Could you check a few things on this model? Use its own coordinates, in mm. Face numbers are marked on the shaded views. A direction names the side the tool comes from. Give positions to 0.01 mm unless a question says otherwise; leave off trailing zeros. Order: outer loops, then holes, each group sorted by start corner. A loop starts at its lowest first (then second) coordinate and runs counter-clockwise, first axis right, second up. Notation, with made-up numbers: (-38, 69) -> (-17, 69) arc R12 ccw to (-17, 83) -> close; hole circle Ø6 at (72, 45). An arc over 180 degrees is marked (long way). One line per item, written item: value.
```python
from build123d import *

# Parameters (mm, degrees)
ESQUISSE1_R                  = 20
EXTRUSION1_DEPTH             = 10.8
ESQUISSE2_R                  = 12
EXTRUSION2_DEPTH             = 15.7
ESQUISSE3_R                  = 11
EXTRUSION3_DEPTH             = 18
CHANFREIN1_SIZE              = 1
CHANFREIN1_OF_SYM_TRIE2_SIZE = 1


with BuildPart() as part:
    # Esquisse1 → Extrusion1 (new, symmetric)
    with BuildSketch(Plane.XY):
        with Locations(Location((0, 0, 0), (0, 0, 180))):
            Circle(ESQUISSE1_R)
    extrude(amount=EXTRUSION1_DEPTH, both=True)

    # Esquisse2 → Extrusion2 (add)
    with BuildSketch(Plane.XY.offset(10.8)):
        with Locations((0, 6.5)):
            Circle(ESQUISSE2_R)
    extrusion2 = extrude(amount=EXTRUSION2_DEPTH)

    # Esquisse3 → Extrusion3 (add)
    with BuildSketch(Plane.XY.offset(26.5)):
        with Locations(Location((0, 10, 0), (0, 0, 171.974698192))):
            Circle(ESQUISSE3_R)
    extrusion3 = extrude(amount=EXTRUSION3_DEPTH)

    # Chanfrein1
    chanfrein1_edges = [part.edges().sort_by_distance(p)[0] for p in [
        (10.892271647, 8.464285714, 44.5),
    ]]
    chamfer(chanfrein1_edges, length=CHANFREIN1_SIZE)

    # Symétrie2: Extrusion2, Extrusion3 across plane
    add(extrusion2.mirror(Plane.XY))
    add(extrusion3.mirror(Plane.XY))

    # Chanfrein1 of Symétrie2
    chanfrein1_of_sym_trie2_edges = [part.edges().sort_by_distance(p)[0] for p in [
        (10.892271647, 8.464285714, -44.5),
    ]]
    chamfer(chanfrein1_of_sym_trie2_edges, length=CHANFREIN1_OF_SYM_TRIE2_SIZE)


solid = part.part
```
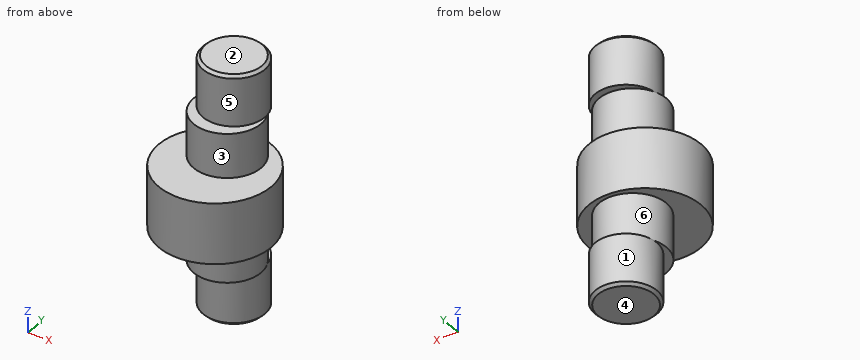
1) If I drill on line 1 along Z through (x, y) = (-6, 17); line 2 along Z through (x, y) = (-5, -12); line 3 along X through (y, z) = (8, -29), over which ranges is the centre line in solid material (lowest first)?
Answer below:
line 1: z = -44.5 to -26.5, -10.8 to 10.8, 26.5 to 44.5
line 2: z = -10.8 to 10.8
line 3: x = -10.82 to 10.82
2) Suppose I cut it at C-C, the plane y = 10. Write out the boundary of the cut face in (x, z).
Answer below:
outline: (-17.32, -10.8) -> (-11.48, -10.8) -> (-11.48, -26.5) -> (-11, -26.5) -> (-11, -43.5) -> (-10, -44.5) -> (10, -44.5) -> (11, -43.5) -> (11, -26.5) -> (11.48, -26.5) -> (11.48, -10.8) -> (17.32, -10.8) -> (17.32, 10.8) -> (11.48, 10.8) -> (11.48, 26.5) -> (11, 26.5) -> (11, 43.5) -> (10, 44.5) -> (-10, 44.5) -> (-11, 43.5) -> (-11, 26.5) -> (-11.48, 26.5) -> (-11.48, 10.8) -> (-17.32, 10.8) -> close
3) For P1, Ø5, axis at x = 10.5, z = -12, coming from the -Y side; P2, Ø10, axis at x = -15.5, y = -14, coming from the +Z side; P3, Ø3, axis at x = -2.5, y = -4, coming from the +Z side, each with a flat end and sliding along its axis, tell me the tip position at first contact or that it passes through.
Answer below:
P1: stops at y = -18.19
P2: stops at z = 10.8
P3: stops at z = 26.5
4) Suppose I cut it at D-D, the plane z = -1. Write out the boundary of the cut face in (x, y).
Answer below:
outline: circle Ø40 at (0, 0)
5) For the marked faces 5 and 6, which set-ups out of +Z, -Z, +X, -X, +Y, -Y let a thin tool reach every point of the face, with its end or its side?
Answer below:
face 5: +Z
face 6: none
6) Suppose I cut it at B-B, the plane z = -33. Write out the boundary of the cut face in (x, y).
Answer below:
outline: circle Ø22 at (0, 10)
7) Suppose I cut it at A-A, the plane x = 0. Write out the boundary of the cut face in (y, z), then the cut area to 3 significant figures.
Answer below:
outline: (-20, -10.8) -> (-5.5, -10.8) -> (-5.5, -26.5) -> (-1, -26.5) -> (-1, -43.5) -> (0, -44.5) -> (20, -44.5) -> (21, -43.5) -> (21, -26.5) -> (18.5, -26.5) -> (18.5, -10.8) -> (20, -10.8) -> (20, 10.8) -> (18.5, 10.8) -> (18.5, 26.5) -> (21, 26.5) -> (21, 43.5) -> (20, 44.5) -> (0, 44.5) -> (-1, 43.5) -> (-1, 26.5) -> (-5.5, 26.5) -> (-5.5, 10.8) -> (-20, 10.8) -> close
area: 2,410 mm2
8) We'd pull the mould along Z, two halves only. Please class the marked faces 1, 2, 3 and 4: +Z half, -Z half, draft (parallel to the pull), parting line (faces both ways), or undercut.
Answer below:
face 1: draft
face 2: +Z half
face 3: undercut
face 4: -Z half
